For this review, take the finished solid that the model builds, in its own axes (mm). A direction names the side the tool comes from. Round coordinates to 2 decimals unless told otherwise and drop trailing zeros. Order: outer loops, then holes, each group sorted by start corner. A loop starts at its lowest first (then second) coordinate and runs counter-clockwise, first axis right, second up. Notation, with made-up numbers: M -9,17.5 L 3,17.5 A23 cw 3,55.5 Z; hole C 31,62 d4. An arc over 180 degrees is marked long. Put each result on its own line as item: value.
from build123d import *

# Parameters (mm, degrees)
SKETCH1_W           = 38.1
SKETCH1_H           = 12.7
BOSS_EXTRUDE1_DEPTH = 10.16
CUT_EXTRUDE1_DEPTH  = 10.16


with BuildPart() as part:
    # Sketch1 → Boss-Extrude1 (new body)
    with BuildSketch(Plane.YZ):
        with Locations((19.05, 6.35)):
            Rectangle(SKETCH1_W, SKETCH1_H)
    extrude(amount=BOSS_EXTRUDE1_DEPTH)

    # Sketch2 → Cut-Extrude1 (cut)
    with BuildSketch(Plane.YZ.offset(10.16)):
        Polygon((2.54, 10.16), (35.56, 10.16), (35.56, 2.621943929), (30.48, 2.621943929), (30.48, 0), (7.656390435, 0), (7.656390435, 2.621943929), (2.54, 2.621943929), align=None)
    extrude(amount=-CUT_EXTRUDE1_DEPTH, mode=Mode.SUBTRACT)


solid = part.part
(1) Add section B-B on y = 32.5. Give the boundary of the cut face in (x, z).
A:
outline: M 0,0 L 10.16,0 L 10.16,2.62 L 0,2.62 Z; M 0,10.16 L 10.16,10.16 L 10.16,12.7 L 0,12.7 Z
(2) To check wall thickness, follow L1, parallel to Y at x = 3, z = 9.25; L2, parallel to Z at x = 2.25, y = 4; L3, parallel to Z at x = 4, y = 15.5. State the ranges of each line that lie inside material, in increasing order.
A:
L1: y = 0 to 2.54, 35.56 to 38.1
L2: z = 0 to 2.62, 10.16 to 12.7
L3: z = 10.16 to 12.7
(3) Add section D-D on y = 13. Give the boundary of the cut face in (x, z).
A:
outline: M 0,10.16 L 10.16,10.16 L 10.16,12.7 L 0,12.7 Z
(4) For faces 1 (the face through (5, 30.48, 1)), 2 (the face through (5, 35.56, 6)), 3 (the face through (10.16, 19, 11)), list the 3-axis set-ups (+Z, -Z, +X, -X, +Y, -Y) from which the entire face can be reached by the end or side of a thin tool; tool diameter is ignored.
A:
face 1: -Z, +X, -X
face 2: +X, -X
face 3: +Z, -Z, +X, +Y, -Y
(5) Add section A-A on z = 2. Give the boundary of the cut face in (x, y), then the cut area to 3 significant figures.
A:
outline: M 0,0 L 10.16,0 L 10.16,7.66 L 0,7.66 Z; M 0,30.48 L 10.16,30.48 L 10.16,38.1 L 0,38.1 Z
area: 155 mm2
(6) Add section C-C on x = 2.5. Give the boundary of the cut face in (y, z), then the cut area to 3 significant figures.
A:
outline: M 0,0 L 7.66,0 L 7.66,2.62 L 2.54,2.62 L 2.54,10.16 L 35.56,10.16 L 35.56,2.62 L 30.48,2.62 L 30.48,0 L 38.1,0 L 38.1,12.7 L 0,12.7 Z
area: 175 mm2
(7) Insertion check: pin 1 Ø1 at (x, z) = (7, 5) entering from -Y; pin 2 Ø1 at (y, z) = (29.5, 8.5) entering from +X. Each pin has a flat end and moves straight along its axis. Give the tip position at first contact, or say it passes through.
A:
pin 1: stops at y = 0
pin 2: passes through
